Geometry: final body of the model. Coordinates: model frame, mm. Face numbers are marked on the shaded views. A direction names the side the tool comes from. Coordinates: 2 decimals unless noted, no trailing zeros. Write each loop counter-clockwise with the first axis right and the second up, starting at its lowest first coordinate (ties: lowest second). Pieces come first, ordered by that corner, then holes. Notation, with made-up numbers: M 65.25,-38.75 L 99.25,-38.75 A13 ccw 99.25,-25.75 Z; hole C 42.25,61 d4. An arc over 180 degrees is marked long. Write item = value, one per line. Start each with the question number.
Item 1: Pull-direction query (Z, two-part tool) for the marked faces 5, 6 and 7; classes: +Z half, -Z half, draft (parallel to the pull), parting line (faces both ways), or undercut.
Item 2: Ray query, L1, parallel to Z at x = 18, y = 264.5; L2, parallel to Z at x = 11.25, y = 284.5; L3, parallel to Z at x = 2, y = 302.5. Return the intervals inside material, ascending. Write a range as [from, to].
Item 3: Section A-A on z = -127. Output: boundary loops of the cut face in (x, y).
Item 4: Section C-C on y = 292. Output: boundary loops of the cut face in (x, z), plus the area to 3 significant figures.
Item 5: Section D-D on z = -99.5. Output: boundary loops of the cut face in (x, y), plus the area to 3 significant figures.
Item 6: Reachability of the marked faces 1, 2, 3 and 4 from +Z, -Z, +X, -X, +Y, -Y: full face, straight path, thin tool, end or side. Return the list, or none.
Item 7: First-contact query: pin 1 Ø8 at (x, y) = (7, 279) entering from +Z; pin 2 Ø3 at (x, y) = (16.5, 308) entering from -Z; pin 3 Ø0.5 at (x, z) = (19.5, -102.5) entering from -Y. Flat tips, straight axial feed; report the tip coordinate or a pass-through.
Item 8: Section B-B on y = 272. Output: boundary loops of the cut face in (x, z).
from build123d import *

# Parameters (mm, degrees)
SKETCH_2_W          = 12
SKETCH_2_H          = 12
SKETCH_2_W_2        = 43
SKETCH_2_H_2        = 23
EXTRUDE_1_DEPTH     = 20
SKETCH_3_W          = 86.114957356
SKETCH_3_H          = 19.725477411
EXTRUDE_2_DEPTH     = 19
CUT_EXTRUDE_1_DEPTH = 18
CUT_EXTRUDE_2_DEPTH = 17


with BuildPart() as part:
    # 草图2 → 凸台-拉伸1 (new body)
    with BuildSketch(Plane(origin=(0, 0, 0), x_dir=(0, 0, -1), z_dir=(1, 0, 0))):
        Polygon((109.86010867, 259.687677289), (122.86010867, 259.687677289), (122.86010867, 287.687677289), (148.86010867, 287.687677289), (148.86010867, 259.687677289), (161.86010867, 259.687677289), (161.86010867, 287.687677289), (175.36010867, 287.687677289), (175.36010867, 259.687677289), (187.36010867, 259.687677289), (187.36010867, 311.687677289), (212.36010867, 311.687677289), (212.36010867, 337.187677289), (187.36010867, 337.187677289), (187.36010867, 361.187677289), (84.36010867, 361.187677289), (84.36010867, 337.187677289), (59.36010867, 337.187677289), (59.36010867, 311.687677289), (84.36010867, 311.687677289), (84.36010867, 259.687677289), (96.36010867, 259.687677289), (96.36010867, 287.687677289), (109.86010867, 287.687677289), align=None)
        with Locations((103.86010867, 343.187677289)):
            Rectangle(SKETCH_2_W, SKETCH_2_H, mode=Mode.SUBTRACT)
        with Locations((135.86010867, 309.687677289)):
            Rectangle(SKETCH_2_W_2, SKETCH_2_H_2, mode=Mode.SUBTRACT)
        with Locations((167.86010867, 343.187677289)):
            Rectangle(SKETCH_2_W, SKETCH_2_H, mode=Mode.SUBTRACT)
    extrude(amount=EXTRUDE_1_DEPTH)

    # 草图3 → 凸台-拉伸2 (add)
    with BuildSketch(Plane.ZY):
        with Locations((-135.786506142, 344.147634955)):
            Rectangle(SKETCH_3_W, SKETCH_3_H)
    extrude(amount=-EXTRUDE_2_DEPTH)

    # 草图4 → 切除-拉伸1 (cut)
    with BuildSketch(Plane.ZY):
        Polygon((-170.36010867, 323.937677289), (-163.36010867, 323.937677289), (-163.36010867, 322.487677289), (-162.36010867, 322.487677289), (-162.36010867, 323.937677289), (-111.36010867, 323.937677289), (-111.36010867, 322.487677289), (-110.36010867, 322.487677289), (-110.36010867, 323.937677289), (-103.36010867, 323.937677289), (-103.36010867, 295.437677289), (-110.36010867, 295.437677289), (-110.36010867, 296.887677289), (-111.36010867, 296.887677289), (-111.36010867, 295.437677289), (-162.36010867, 295.437677289), (-162.36010867, 296.887677289), (-163.36010867, 296.887677289), (-163.36010867, 295.437677289), (-170.36010867, 295.437677289), align=None)
    extrude(amount=-CUT_EXTRUDE_1_DEPTH, mode=Mode.SUBTRACT)

    # 草图5 → 切除-拉伸2 (cut)
    with BuildSketch(Plane.ZY):
        Polygon((-192.36010867, 316.687677289), (-157.36010867, 316.687677289), (-157.36010867, 302.687677289), (-177.960754488, 302.687677289), (-177.960754488, 259.687677289), (-184.732187032, 259.687677289), (-184.732187032, 302.687677289), (-192.36010867, 302.687677289), align=None)
    extrude(amount=-CUT_EXTRUDE_2_DEPTH, mode=Mode.SUBTRACT)


solid = part.part
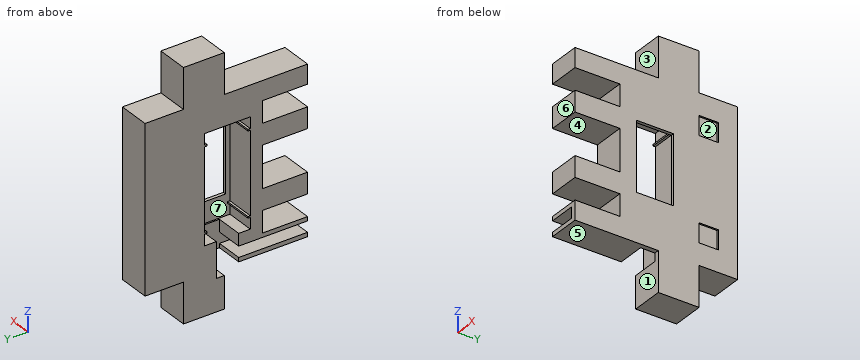
Responses:
q1.face_5 = -Z half
q1.face_6 = draft
q1.face_7 = undercut
q2.L1 = [-187.36, -175.36], [-161.86, -148.86], [-122.86, -109.86], [-96.36, -84.36]
q2.L2 = [-187.36, -184.73], [-177.96, -175.36], [-161.86, -148.86], [-122.86, -109.86], [-96.36, -84.36]
q2.L3 = [-187.36, -184.73], [-177.96, -170.36], [-103.36, -84.36]
q3.outline = M 0,287.69 L 20,287.69 L 20,298.19 L 18,298.19 L 18,295.44 L 0,295.44 Z; M 0,323.94 L 18,323.94 L 18,321.19 L 20,321.19 L 20,361.19 L 0,361.19 Z
q4.outline = M 0,-187.36 L 20,-187.36 L 20,-84.36 L 0,-84.36 L 0,-177.96 L 17,-177.96 L 17,-184.73 L 0,-184.73 Z
q4.area = 1,940 mm²
q5.outline = M 0,287.69 L 20,287.69 L 20,337.19 L 19,337.19 L 19,349.19 L 20,349.19 L 20,361.19 L 0,361.19 Z
q5.area = 1,460 mm²
q6.face_1 = -Z, +X, -X, -Y
q6.face_2 = +X
q6.face_3 = +Z, +X, -X, -Y
q6.face_4 = +X, -X, -Y
q7.pin_1 = -84.36
q7.pin_2 = -187.36
q7.pin_3 = 287.69
q8.outline = M 0,-187.36 L 20,-187.36 L 20,-175.36 L 0,-175.36 L 0,-177.96 L 17,-177.96 L 17,-184.73 L 0,-184.73 Z; M 0,-161.86 L 20,-161.86 L 20,-148.86 L 0,-148.86 Z; M 0,-122.86 L 20,-122.86 L 20,-109.86 L 0,-109.86 Z; M 0,-96.36 L 20,-96.36 L 20,-84.36 L 0,-84.36 Z
